Read the model definition and answer for the solid it produces. Units are mm, in the model's axes. Coordinates: 2 decimals unless noted, no trailing zeros. Order: outer loops, then holes, each group sorted by start corner. A loop starts at its lowest first (then second) coordinate and runs counter-clockwise, first axis right, second up.
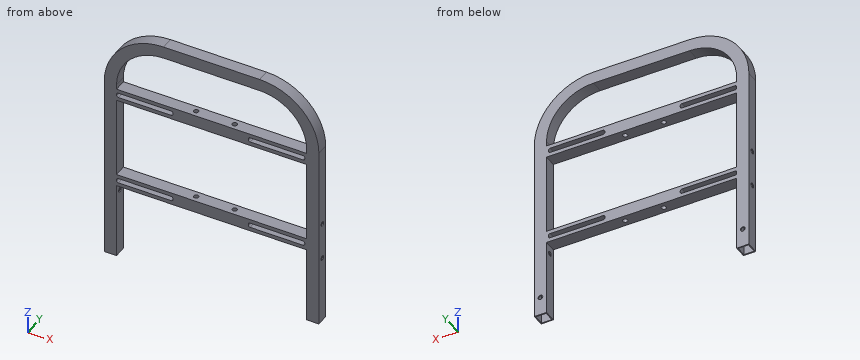
```python
from build123d import *

# Parameters (mm, degrees)
BOSS_EXTRUDE1_DEPTH = 33.02
BOSS_EXTRUDE2_REACH = 840.177
SKETCH3_W           = 33.02
SKETCH3_H           = 33.02
CUT_EXTRUDE1_DEPTH  = 699.684702852
CUT_EXTRUDE2_REACH  = 548.478
SKETCH6_R           = 6.35
LPATTERN1_COUNT     = 2
LPATTERN1_PITCH     = 254
SHELL1_T            = -2.54
CUT_EXTRUDE3_REACH  = 730.825
SKETCH7_W           = 27.94
SKETCH7_H           = 27.94
CUT_EXTRUDE4_REACH  = 700.685
SKETCH8_R           = 6.35
CUT_EXTRUDE5_REACH  = 862.055
SKETCH9_R           = 6.35
CUT_EXTRUDE6_REACH  = 862.055
SKETCH10_R          = 6.35
SKETCH15_R          = 6.35
CUT_EXTRUDE10_DEPTH = 839.176908773
SKETCH16_R          = 6.35
CUT_EXTRUDE11_DEPTH = 861.055402169


with BuildPart() as part:
    # Sketch1 → Boss-Extrude1 (new body)
    with BuildSketch(Plane(origin=(0, 0, 0), x_dir=(1, 0, 0), z_dir=(0, 1, 0))):
        with BuildLine():
            Line((-256.54, 635), (-256.54, 127))
            ThreePointArc((-256.54, 127), (-219.342561211, 37.197438789), (-129.54, 0))
            Line((-129.54, 0), (129.54, 0))
            ThreePointArc((129.54, 0), (219.342561211, 37.197438789), (256.54, 127))
            Line((256.54, 127), (256.54, 635))
            Line((256.54, 635), (289.56, 635))
            Line((289.56, 635), (289.56, 127))
            ThreePointArc((289.56, 127), (242.691227125, 13.848772875), (129.54, -33.02))
            Line((129.54, -33.02), (-129.54, -33.02))
            ThreePointArc((-129.54, -33.02), (-242.691227125, 13.848772875), (-289.56, 127))
            Line((-289.56, 127), (-289.56, 635))
            Line((-289.56, 635), (-256.54, 635))
        make_face()
    extrude(amount=-BOSS_EXTRUDE1_DEPTH)

    # Sketch3 → Boss-Extrude2 (add, up to next)
    with BuildSketch(Plane(origin=(-256.54, 0, 0), x_dir=(0, 0, -1), z_dir=(1, 0, 0)), mode=Mode.PRIVATE) as boss_extrude2_sk1:
        with Locations((156.21, -16.51)):
            Rectangle(SKETCH3_W, SKETCH3_H)
    boss_extrude2_tool1 = extrude(boss_extrude2_sk1.sketch, amount=BOSS_EXTRUDE2_REACH, mode=Mode.PRIVATE) - part.part
    boss_extrude2 = boss_extrude2_tool1.solids().sort_by_distance((-256.54, -16.51, -156.21))[0]
    add(boss_extrude2)

    # Sketch5 → Cut-Extrude1 (cut, through all)
    with BuildSketch(Plane(origin=(0, 0, 0), x_dir=(1, 0, 0), z_dir=(0, 1, 0))):
        with BuildLine():
            Line((-251.46, 162.56), (-109.22, 162.56))
            ThreePointArc((-109.22, 162.56), (-105.627897552, 161.072102448), (-104.14, 157.48))
            Line((-104.14, 157.48), (-104.14, 154.94))
            ThreePointArc((-104.14, 154.94), (-105.627897552, 151.347897552), (-109.22, 149.86))
            Line((-109.22, 149.86), (-251.46, 149.86))
            ThreePointArc((-251.46, 149.86), (-255.052102448, 151.347897552), (-256.54, 154.94))
            Line((-256.54, 154.94), (-256.54, 157.48))
            ThreePointArc((-256.54, 157.48), (-255.052102448, 161.072102448), (-251.46, 162.56))
        make_face()
        with BuildLine():
            Line((99.06, 157.48), (99.06, 154.94))
            ThreePointArc((99.06, 154.94), (100.547897552, 151.347897552), (104.14, 149.86))
            Line((104.14, 149.86), (246.38, 149.86))
            ThreePointArc((246.38, 149.86), (249.972102448, 151.347897552), (251.46, 154.94))
            Line((251.46, 154.94), (251.46, 157.48))
            ThreePointArc((251.46, 157.48), (249.972102448, 161.072102448), (246.38, 162.56))
            Line((246.38, 162.56), (104.14, 162.56))
            ThreePointArc((104.14, 162.56), (100.547897552, 161.072102448), (99.06, 157.48))
        make_face()
    cut_extrude1 = extrude(amount=-CUT_EXTRUDE1_DEPTH, mode=Mode.SUBTRACT)

    # Sketch6 → Cut-Extrude2 (cut, up to next)
    with BuildSketch(Plane(origin=(0, 0, -172.72), x_dir=(-1, 0, 0), z_dir=(0, 0, -1)), mode=Mode.PRIVATE) as cut_extrude2_sk1:
        with Locations(Location((50.8, -16.51, 0), (0, 0, 90))):
            Circle(SKETCH6_R)
    cut_extrude2_tool1 = extrude(cut_extrude2_sk1.sketch, amount=-CUT_EXTRUDE2_REACH, mode=Mode.PRIVATE) & part.part
    # Sketch6 → Cut-Extrude2 (cut, up to next)
    with BuildSketch(Plane(origin=(0, 0, -172.72), x_dir=(-1, 0, 0), z_dir=(0, 0, -1)), mode=Mode.PRIVATE) as cut_extrude2_sk2:
        with Locations(Location((-53.34, -16.51, 0), (0, 0, 90))):
            Circle(SKETCH6_R)
    cut_extrude2_tool2 = extrude(cut_extrude2_sk2.sketch, amount=-CUT_EXTRUDE2_REACH, mode=Mode.PRIVATE) & part.part
    cut_extrude2_1 = cut_extrude2_tool1.solids().sort_by_distance((-50.8, -16.51, -172.72))[0]
    add(cut_extrude2_1, mode=Mode.SUBTRACT)
    cut_extrude2_2 = cut_extrude2_tool2.solids().sort_by_distance((53.34, -16.51, -172.72))[0]
    add(cut_extrude2_2, mode=Mode.SUBTRACT)
    cut_extrude2 = cut_extrude2_1 + cut_extrude2_2  # Cut-Extrude2 as one shape, for the pattern or mirror that repeats it

    # LPattern1: Boss-Extrude2, Cut-Extrude1, Cut-Extrude2 ×2
    with Locations(*[(0, 0, -i * LPATTERN1_PITCH) for i in range(1, LPATTERN1_COUNT)]):
        add(boss_extrude2)
        add(cut_extrude1, mode=Mode.SUBTRACT)
        add(cut_extrude2, mode=Mode.SUBTRACT)

    # Shell1
    shell1_openings = [part.faces().sort_by_distance(p)[0] for p in [
        (273.05, -16.51, -635),
    ]]
    offset(amount=SHELL1_T, openings=shell1_openings, kind=Kind.INTERSECTION)

    # Sketch7 → Cut-Extrude3 (cut, up to next)
    with BuildSketch(Plane(origin=(0, 0, -635), x_dir=(-1, 0, 0), z_dir=(0, 0, -1)), mode=Mode.PRIVATE) as cut_extrude3_sk1:
        with Locations((273.05, -16.51)):
            Rectangle(SKETCH7_W, SKETCH7_H)
    cut_extrude3_tool1 = extrude(cut_extrude3_sk1.sketch, amount=-CUT_EXTRUDE3_REACH, mode=Mode.PRIVATE) & part.part
    add(cut_extrude3_tool1.solids().sort_by_distance((-273.05, -16.51, -635))[0], mode=Mode.SUBTRACT)

    # Sketch8 → Cut-Extrude4 (cut, up to next)
    with BuildSketch(Plane(origin=(0, 0, 0), x_dir=(1, 0, 0), z_dir=(0, 1, 0)), mode=Mode.PRIVATE) as cut_extrude4_sk1:
        with Locations(Location((-273.05, 584.2, 0), (0, 0, 270))):
            Circle(SKETCH8_R)
    cut_extrude4_tool1 = extrude(cut_extrude4_sk1.sketch, amount=-CUT_EXTRUDE4_REACH, mode=Mode.PRIVATE) & part.part
    # Sketch8 → Cut-Extrude4 (cut, up to next)
    with BuildSketch(Plane(origin=(0, 0, 0), x_dir=(1, 0, 0), z_dir=(0, 1, 0)), mode=Mode.PRIVATE) as cut_extrude4_sk2:
        with Locations(Location((273.05, 584.2, 0), (0, 0, 270))):
            Circle(SKETCH8_R)
    cut_extrude4_tool2 = extrude(cut_extrude4_sk2.sketch, amount=-CUT_EXTRUDE4_REACH, mode=Mode.PRIVATE) & part.part
    add(cut_extrude4_tool1.solids().sort_by_distance((-273.05, 0, -584.2))[0], mode=Mode.SUBTRACT)
    add(cut_extrude4_tool2.solids().sort_by_distance((273.05, 0, -584.2))[0], mode=Mode.SUBTRACT)

    # Sketch9 → Cut-Extrude5 (cut, up to next)
    with BuildSketch(Plane(origin=(289.56, 0, 0), x_dir=(0, 0, -1), z_dir=(1, 0, 0)), mode=Mode.PRIVATE) as cut_extrude5_sk1:
        with Locations((347.98, -16.51)):
            Circle(SKETCH9_R)
    cut_extrude5_tool1 = extrude(cut_extrude5_sk1.sketch, amount=-CUT_EXTRUDE5_REACH, mode=Mode.PRIVATE) & part.part
    # Sketch9 → Cut-Extrude5 (cut, up to next)
    with BuildSketch(Plane(origin=(289.56, 0, 0), x_dir=(0, 0, -1), z_dir=(1, 0, 0)), mode=Mode.PRIVATE) as cut_extrude5_sk2:
        with Locations((449.58, -16.51)):
            Circle(SKETCH9_R)
    cut_extrude5_tool2 = extrude(cut_extrude5_sk2.sketch, amount=-CUT_EXTRUDE5_REACH, mode=Mode.PRIVATE) & part.part
    add(cut_extrude5_tool1.solids().sort_by_distance((289.56, -16.51, -347.98))[0], mode=Mode.SUBTRACT)
    add(cut_extrude5_tool2.solids().sort_by_distance((289.56, -16.51, -449.58))[0], mode=Mode.SUBTRACT)

    # Sketch10 → Cut-Extrude6 (cut, up to next)
    with BuildSketch(Plane.ZY.offset(289.56), mode=Mode.PRIVATE) as cut_extrude6_sk1:
        with Locations(Location((-347.98, -16.51, 0), (0, 0, 180))):
            Circle(SKETCH10_R)
    cut_extrude6_tool1 = extrude(cut_extrude6_sk1.sketch, amount=-CUT_EXTRUDE6_REACH, mode=Mode.PRIVATE) & part.part
    add(cut_extrude6_tool1.solids().sort_by_distance((-289.56, -16.51, -347.98))[0], mode=Mode.SUBTRACT)

    # Sketch15 → Cut-Extrude10 (cut, through all)
    with BuildSketch(Plane.ZY.offset(-256.54)):
        with Locations(Location((-449.58, -16.51, 0), (0, 0, 180))):
            Circle(SKETCH15_R)
    extrude(amount=-CUT_EXTRUDE10_DEPTH, mode=Mode.SUBTRACT)

    # Sketch16 → Cut-Extrude11 (cut, through all)
    with BuildSketch(Plane.ZY.offset(289.56)):
        with Locations(Location((-449.58, -16.51, 0), (0, 0, 180))):
            Circle(SKETCH16_R)
    extrude(amount=-CUT_EXTRUDE11_DEPTH, mode=Mode.SUBTRACT)


solid = part.part
```
1) A cutting plane is placed at A-A, the plane x = 77.5. Determine the outline of the cut face in (y, z), and give its area (3 significant figures).
A:
outline: (-33.02, -426.72) - (0, -426.72) - (0, -393.7) - (-33.02, -393.7) - close; (-33.02, -172.72) - (0, -172.72) - (0, -139.7) - (-33.02, -139.7) - close; (-33.02, 0) - (0, 0) - (0, 33.02) - (-33.02, 33.02) - close; hole (-30.48, -424.18) - (-2.54, -424.18) - (-2.54, -396.24) - (-30.48, -396.24) - close; hole (-30.48, -170.18) - (-2.54, -170.18) - (-2.54, -142.24) - (-30.48, -142.24) - close; hole (-30.48, 2.54) - (-2.54, 2.54) - (-2.54, 30.48) - (-30.48, 30.48) - close
area: 929 mm2
2) Flat-ended cylindrical pins translate along their axes: pin 1 Ø10 at (x, y) = (-50.8, -16.51) entering from -Z; pin 2 Ø10 at (x, y) = (-71.5, -10) entering from -Z; pin 3 Ø2 at (y, z) = (-7, -109) entering from +X; pin 4 Ø10 at (y, z) = (-16.51, -449.58) entering from -X. Find the tip coordinate at first contact, or state that the pin passes through.
A:
pin 1: stops at z = 0
pin 2: stops at z = -426.72
pin 3: stops at x = 288.65
pin 4: passes through
3) A cutting plane is placed at C-C, the plane y = -16.51. State how many separate pieces and enclosed holes the cut face has, and give its area (3 significant figures).
A:
separate pieces: 14
enclosed holes: 6
area: 17,200 mm2
4) Straight lines are drawn through the part: line 1 (X direction, y = -29, z = -284); line 2 (Z direction, x = -9, y = -9); line 3 (Y direction, x = 19.5, z = -167). For each, find the intervals that lie inside material, in ascending order.
A:
line 1: x = -289.56 to -287.02, -259.08 to -256.54, 256.54 to 259.08, 287.02 to 289.56
line 2: z = -426.72 to -424.18, -396.24 to -393.7, -172.72 to -170.18, -142.24 to -139.7, 0 to 2.54, 30.48 to 33.02
line 3: y = -33.02 to -30.48, -2.54 to 0
5) A cutting plane is placed at B-B, the plane z = -566.5. Determine the outline of the cut face in (x, y).
A:
outline: (-289.56, -33.02) - (-256.54, -33.02) - (-256.54, 0) - (-289.56, 0) - close; (256.54, -33.02) - (289.56, -33.02) - (289.56, 0) - (256.54, 0) - close; hole (-287.02, -30.48) - (-259.08, -30.48) - (-259.08, -2.54) - (-287.02, -2.54) - close; hole (259.08, -30.48) - (287.02, -30.48) - (287.02, -2.54) - (259.08, -2.54) - close
